Geometry check sheet. Reference: the model listing, model coordinates, mm. Face numbers are marked on the shaded views. Round coordinates to 2 decimals unless told otherwise and drop trailing zeros. Write each loop counter-clockwise with the first axis right and the second up, starting at its lowest first coordinate (ties: lowest second). Pieces come first, ordered by that corner, then holes. Notation, with made-up numbers: (44.25, 75) -> (100.25, 75) arc R22 cw to (100.25, 88) -> close; hole circle Ø6 at (87, 81). An arc over 180 degrees is marked (long way). Use a Markdown table: item, result.
```python
from build123d import *

# Parameters (mm, degrees)
F2_DEPTH  = 6
F3_T      = -0.75
F4_R      = 1
F5_DEPTH  = 6
F6_W      = 13.25
F6_H      = 5.25
F6_W_2    = 7.5
F7_DEPTH  = 0.75
F9_DEPTH  = 4
F10_W     = 12.9
F10_H     = 5
F11_DEPTH = 1
F12_R     = 2
F13_DEPTH = 4
F14_W     = 53
F14_H     = 53
F15_DEPTH = 3
F16_R     = 1
F17_R     = 5
F18_W     = 4
F18_H     = 2.5
F19_DEPTH = 1.5


with BuildPart() as f2:
    # F1 (on Top) → F2 (new body)
    with BuildSketch(Plane.XY):
        Polygon((-28.45, 16.95), (-28.45, -16.95), (28.45, -16.95), (28.45, 16.95), (16.2, 16.95), (1.45, 16.95), (-9.05, 16.95), (-18.3, 16.95), align=None)
    extrude(amount=F2_DEPTH)

    # F3
    f3_openings = [f2.faces().sort_by_distance(p)[0] for p in [
        (0, 0, 6),
    ]]
    offset(amount=F3_T, openings=f3_openings)

    # F4 (on Top) → F5 (join)
    with BuildSketch(Plane.XY):
        with Locations((-24.025, 12.525)):
            Circle(F4_R)
        with Locations((24.025, 12.525)):
            Circle(F4_R)
        with Locations((-24.025, -14.025)):
            Circle(F4_R)
        with Locations((24.025, -14.025)):
            Circle(F4_R)
    extrude(amount=F5_DEPTH)

    # F6 (on face) → F7 (cut)
    with BuildSketch(Plane(origin=(0, 16.95, 0), x_dir=(-1, 0, 0), z_dir=(0, 1, 0))):
        with Locations((-8.875, 3.375)):
            Rectangle(F6_W, F6_H)
        with Locations((13.75, 3.375)):
            Rectangle(F6_W_2, F6_H)
    extrude(amount=-F7_DEPTH, mode=Mode.SUBTRACT)

    # F8 (on face) → F9 (join)
    with BuildSketch(Plane(origin=(0, 0, 0), x_dir=(1, 0, 0), z_dir=(0, 0, -1))):
        with BuildLine():
            ThreePointArc((-28.5, 24), (-25.6715728753, 25.1715728753), (-24.5, 28))
            Line((-24.5, 28), (-28.5, 28))
            Line((-28.5, 28), (-28.5, 24))
        make_face()
        with BuildLine():
            Line((-28.5, 28), (-24.5, 28))
            ThreePointArc((-24.5, 28), (-31.3284271247, 30.8284271247), (-28.5, 24))
            Line((-28.5, 24), (-28.5, 28))
        make_face()
        with BuildLine():
            Line((24.5, 28), (-24.5, 28))
            ThreePointArc((-24.5, 28), (-25.6715728753, 25.1715728753), (-28.5, 24))
            Line((-28.5, 24), (-28.5, -24))
            ThreePointArc((-28.5, -24), (-25.6715728753, -25.1715728753), (-24.5, -28))
            Line((-24.5, -28), (24.5, -28))
            ThreePointArc((24.5, -28), (25.6715728753, -25.1715728753), (28.5, -24))
            Line((28.5, -24), (28.5, 24))
            ThreePointArc((28.5, 24), (25.6715728753, 25.1715728753), (24.5, 28))
        make_face()
        with BuildLine():
            ThreePointArc((32.5, 28), (28.5, 32), (24.5, 28))
            Line((24.5, 28), (28.5, 28))
            Line((28.5, 28), (28.5, 24))
            ThreePointArc((28.5, 24), (31.3284271247, 25.1715728753), (32.5, 28))
        make_face()
        with BuildLine():
            Line((28.5, 28), (24.5, 28))
            ThreePointArc((24.5, 28), (25.6715728753, 25.1715728753), (28.5, 24))
            Line((28.5, 24), (28.5, 28))
        make_face()
        with BuildLine():
            ThreePointArc((-24.5, -28), (-25.6715728753, -25.1715728753), (-28.5, -24))
            Line((-28.5, -24), (-28.5, -28))
            Line((-28.5, -28), (-24.5, -28))
        make_face()
        with BuildLine():
            Line((-28.5, -28), (-28.5, -24))
            ThreePointArc((-28.5, -24), (-31.3284271247, -30.8284271247), (-24.5, -28))
            Line((-24.5, -28), (-28.5, -28))
        make_face()
        with BuildLine():
            ThreePointArc((32.5, -28), (31.3284271247, -25.1715728753), (28.5, -24))
            Line((28.5, -24), (28.5, -28))
            Line((28.5, -28), (24.5, -28))
            ThreePointArc((24.5, -28), (28.5, -32), (32.5, -28))
        make_face()
        with BuildLine():
            Line((28.5, -28), (28.5, -24))
            ThreePointArc((28.5, -24), (25.6715728753, -25.1715728753), (24.5, -28))
            Line((24.5, -28), (28.5, -28))
        make_face()
    extrude(amount=F9_DEPTH)

    # F10 (on face) → F11 (cut)
    with BuildSketch(Plane.XZ.offset(16.95)):
        with Locations((0, 3.5)):
            Rectangle(F10_W, F10_H)
    extrude(amount=-F11_DEPTH, mode=Mode.SUBTRACT)

    # F12 (on face) → F13 (cut, through all)
    with BuildSketch(Plane(origin=(0, 0, -4), x_dir=(1, 0, 0), z_dir=(0, 0, -1))):
        with Locations((-28.5, 28)):
            Circle(F12_R)
        with Locations((28.5, 28)):
            Circle(F12_R)
        with Locations((28.5, -28)):
            Circle(F12_R)
        with Locations((-28.5, -28)):
            Circle(F12_R)
    extrude(amount=-F13_DEPTH, mode=Mode.SUBTRACT)

    # F14 (on face) → F15 (cut)
    with BuildSketch(Plane(origin=(0, 0, -4), x_dir=(1, 0, 0), z_dir=(0, 0, -1))):
        Rectangle(F14_W, F14_H)
    extrude(amount=-F15_DEPTH, mode=Mode.SUBTRACT)

    # F16
    f16_edges = [f2.edges().sort_by_distance(p)[0] for p in [
        (-26.5, -26.5, -2.5),
        (26.5, -26.5, -2.5),
        (26.5, 26.5, -2.5),
        (-26.5, 26.5, -2.5),
    ]]
    fillet(f16_edges, radius=F16_R)

    # F17
    f17_edges = [f2.edges().sort_by_distance(p)[0] for p in [
        (-27.7, 16.2, 3.375),
        (27.7, 16.2, 3.375),
    ]]
    fillet(f17_edges, radius=F17_R)

    # F18 (on face) → F19 (cut, through all)
    with BuildSketch(Plane.XZ.offset(28)):
        with Locations((0, -2.75)):
            Rectangle(F18_W, F18_H)
    extrude(amount=-F19_DEPTH, mode=Mode.SUBTRACT)


solid = f2.part
```
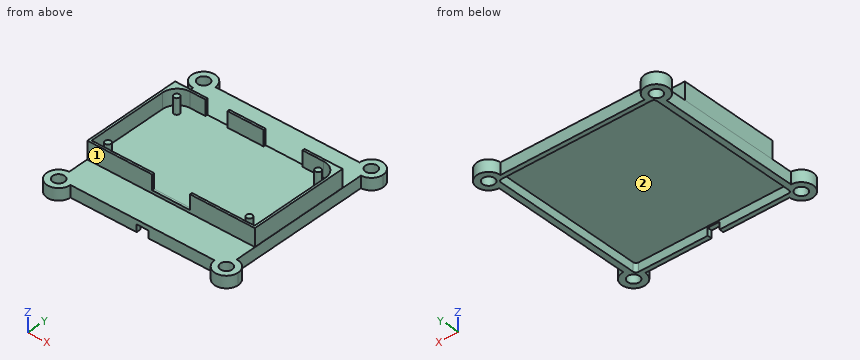
(1) Thickness scan on line 1 (X direction, y = 9.5, z = -2.5); line 2 (X direction, y = -0.5, z = 5.5); line 3 (Y direction, x = -11.5, z = -3). Record the ranges inside material, lowest first.
A:
| item | result |
|---|---|
| line 1 | x = -28.5 to -26.5, 26.5 to 28.5 |
| line 2 | x = -28.45 to -27.7, 27.7 to 28.45 |
| line 3 | y = -28 to -26.5, 26.5 to 28 |
(2) Section check B-B on y = 8. Record the cut outline in (x, z), plus the area to 3 significant figures.
A:
| item | result |
|---|---|
| outline | (-28.5, -4) -> (-26.5, -4) -> (-26.5, -1) -> (26.5, -1) -> (26.5, -4) -> (28.5, -4) -> (28.5, 0) -> (28.45, 0) -> (28.45, 6) -> (27.7, 6) -> (27.7, 0.75) -> (-27.7, 0.75) -> (-27.7, 6) -> (-28.45, 6) -> (-28.45, 0) -> (-28.5, 0) -> close |
| area | 120 mm2 |
(3) Section check C-C on z = 2.25. Record the cut outline in (x, y) (3 decimals).
A:
| item | result |
|---|---|
| outline | (-28.45, -16.95) -> (-6.45, -16.95) -> (-6.45, -16.2) -> (-27.7, -16.2) -> (-27.7, 11.2) arc R5 cw to (-22.7, 16.2) -> (-17.5, 16.2) -> (-17.5, 16.95) -> (-28.45, 16.95) -> close; circle Ø2 at (-24.025, -14.025); circle Ø2 at (-24.025, 12.525); (-10, 16.2) -> (2.25, 16.2) -> (2.25, 16.95) -> (-10, 16.95) -> close; (6.45, -16.95) -> (28.45, -16.95) -> (28.45, 16.95) -> (15.5, 16.95) -> (15.5, 16.2) -> (22.7, 16.2) arc R5 cw to (27.7, 11.2) -> (27.7, -16.2) -> (6.45, -16.2) -> close; circle Ø2 at (24.025, -14.025); circle Ø2 at (24.025, 12.525) |
(4) Section check D-D on x = 17. Record the cut outline in (y, z), plus the area to 3 significant figures.
A:
| item | result |
|---|---|
| outline | (-28, -4) -> (-26.5, -4) -> (-26.5, -1) -> (26.5, -1) -> (26.5, -4) -> (28, -4) -> (28, 0) -> (16.95, 0) -> (16.95, 6) -> (16.2, 6) -> (16.2, 0.75) -> (-16.2, 0.75) -> (-16.2, 6) -> (-16.95, 6) -> (-16.95, 0) -> (-28, 0) -> close |
| area | 98.3 mm2 |
(5) Release check for a two-part mould opening along X. For the marked faces 1 and 2 record: +X half, -X half, draft (parallel to the pull), parting line (faces both ways), or undercut.
A:
| item | result |
|---|---|
| face 1 | draft |
| face 2 | undercut |
(6) Gauge pin test, flat ends, axial feed: pin 1 Ø2 at (x, z) = (-21, 2) entering from -Y; pin 2 Ø3.5 at (x, y) = (28.5, -28) entering from +Z; pin 3 Ø3 at (y, z) = (-5, 4) entering from -X; pin 4 Ø1.2 at (y, z) = (2, -2.5) entering from +X. Record the tip position at first contact, or that the pin passes through.
A:
| item | result |
|---|---|
| pin 1 | stops at y = -16.95 |
| pin 2 | passes through |
| pin 3 | stops at x = -28.45 |
| pin 4 | stops at x = 28.5 |
(7) Section check A-A on z = -2.5. Record the cut outline in (x, y), plus the area to 3 significant figures.
A:
| item | result |
|---|---|
| outline | (-28.5, -24) arc R4 ccw (long way) to (-24.5, -28) -> (-2, -28) -> (-2, -26.5) -> (-25.5, -26.5) arc R1 cw to (-26.5, -25.5) -> (-26.5, 25.5) arc R1 cw to (-25.5, 26.5) -> (25.5, 26.5) arc R1 cw to (26.5, 25.5) -> (26.5, -25.5) arc R1 cw to (25.5, -26.5) -> (2, -26.5) -> (2, -28) -> (24.5, -28) arc R4 ccw (long way) to (28.5, -24) -> (28.5, 24) arc R4 ccw (long way) to (24.5, 28) -> (-24.5, 28) arc R4 ccw (long way) to (-28.5, 24) -> close; hole circle Ø4 at (-28.5, -28); hole circle Ø4 at (-28.5, 28); hole circle Ø4 at (28.5, -28); hole circle Ø4 at (28.5, 28) |
| area | 478 mm2 |
